The model under review builds one solid part; all positions refer to its coordinate system, in mm. Face numbers are marked on the shaded views. A direction names the side the tool comes from. Give positions to 0.01 mm unless a question says otherwise; leave off trailing zeros. Order: outer loops, then holes, each group sorted by start corner. A loop starts at its lowest first (then second) coordinate and runs counter-clockwise, first axis right, second up. Notation, with made-up numbers: (62, 12.5) - (113, 12.5) arc R31 ccw to (113, 41.5) - close; hole circle Ø5 at (50.25, -29). An arc over 180 degrees is marked (long way). Write item = value, one per line. Start each with the question number.
1. We need section B-B, the plane z = 0. Give the boundary of the cut face in (x, y).
2. Machinability: for the marked faces 1 and 2, which of the approach directions +Z, -Z, +X, -X, +Y, -Y give a long, thin tool a straight path to every point of the face, cutting with its end or side? Answer none if there is none.
3. We need section A-A, the plane x = 0. Give the boundary of the cut face in (y, z), and give its area (3 significant figures).
4. Wall thickness on probe 1 along X at (y, z) = (25.5, 0); probe 2 along Y at (x, z) = (-9, -9); probe 3 along X at (y, z) = (4, 15): over which ranges is each line inside the solid? List them lowest first.
5. We need section C-C, the plane y = 27. Give the boundary of the cut face in (x, z).
6. For P1, Ø5.5, axis at x = 0, z = 15, coming from the +Y side; P2, Ø8, axis at y = 18, z = -6.5, coming from the +X side; P3, Ø4, axis at y = 17.5, z = 5.5, coming from the -X side; P4, Ø10, axis at y = 15, z = 2, coming from the +X side, all flat-tipped, find the tip position at first contact; note any pin that passes through.
7. Mouldability with a two-part tool opening along Z and no side actions: class the marked faces 3, 4, 5 and 6 as pulls with the +Z half, pulls with the -Z half, needs draft (parallel to the pull), parting line crosses it, or undercut.
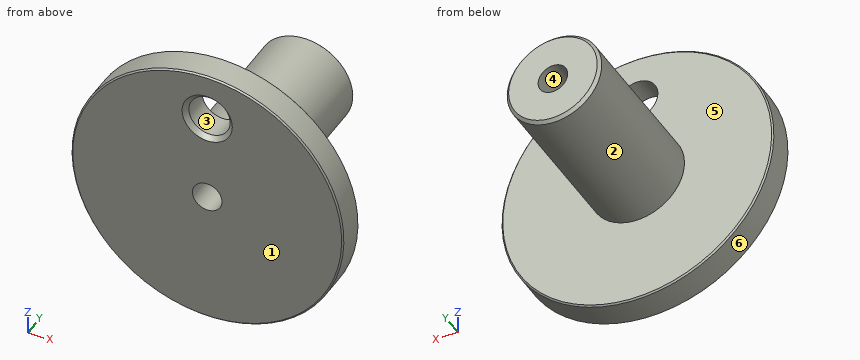
from build123d import *

# Parameters (mm, degrees)
SKETCH1_R           = 23
BOSS_EXTRUDE1_DEPTH = 32
SKETCH2_OUTSIDE_W   = 62.5
SKETCH2_OUTSIDE_H   = 62.5
SKETCH2_OUTSIDE_R   = 8
CUT_EXTRUDE1_DEPTH  = 27
SKETCH3_R           = 2.5
CUT_EXTRUDE2_DEPTH  = 46.628938186
CHAMFER1_SIZE       = 0.5
CHAMFER2_SIZE       = 0.25
SKETCH4_R           = 3.5
CUT_EXTRUDE3_DEPTH  = 46.628938186
CHAMFER3_SIZE       = 0.75


with BuildPart() as part:
    # Sketch1 → Boss-Extrude1 (new body)
    with BuildSketch(Plane(origin=(0, 0, 0), x_dir=(1, 0, 0), z_dir=(0, 1, 0))):
        with Locations(Location((0, 0, 0), (0, 0, 270))):
            Circle(SKETCH1_R)
    extrude(amount=BOSS_EXTRUDE1_DEPTH)

    # Sketch2 outside → Cut-Extrude1 (cut)
    with BuildSketch(Plane(origin=(0, 32, 0), x_dir=(1, 0, 0), z_dir=(0, 1, 0))):
        Rectangle(SKETCH2_OUTSIDE_W, SKETCH2_OUTSIDE_H)
        with Locations(Location((0, 0, 0), (0, 0, 270))):
            Circle(SKETCH2_OUTSIDE_R, mode=Mode.SUBTRACT)
    extrude(amount=-CUT_EXTRUDE1_DEPTH, mode=Mode.SUBTRACT)

    # Sketch3 → Cut-Extrude2 (cut, through all)
    with BuildSketch(Plane(origin=(0, 32, 0), x_dir=(1, 0, 0), z_dir=(0, 1, 0))):
        with Locations(Location((0, 0, 0), (0, 0, 270))):
            Circle(SKETCH3_R)
    extrude(amount=-CUT_EXTRUDE2_DEPTH, mode=Mode.SUBTRACT)

    # Chamfer1
    chamfer1_edges = [part.edges().sort_by_distance(p)[0] for p in [
        (0, 32, -8),
    ]]
    chamfer(chamfer1_edges, length=CHAMFER1_SIZE)

    # Chamfer2
    chamfer2_edges = [part.edges().sort_by_distance(p)[0] for p in [
        (0, 0, -23),
        (0, 5, -23),
    ]]
    chamfer(chamfer2_edges, length=CHAMFER2_SIZE)

    # Sketch4 → Cut-Extrude3 (cut, through all)
    with BuildSketch(Plane.XZ):
        with Locations(Location((0, 15, 0), (0, 0, 270))):
            Circle(SKETCH4_R)
    extrude(amount=-CUT_EXTRUDE3_DEPTH, mode=Mode.SUBTRACT)

    # Chamfer3
    chamfer3_edges = [part.edges().sort_by_distance(p)[0] for p in [
        (0, 0, 18.5),
    ]]
    chamfer(chamfer3_edges, length=CHAMFER3_SIZE)


solid = part.part
Model answer:
q1.outline = (-23, 0.25) - (-22.75, 0) - (-2.5, 0) - (-2.5, 32) - (-7.5, 32) - (-8, 31.5) - (-8, 5) - (-22.75, 5) - (-23, 4.75) - close; (2.5, 0) - (22.75, 0) - (23, 0.25) - (23, 4.75) - (22.75, 5) - (8, 5) - (8, 31.5) - (7.5, 32) - (2.5, 32) - close
q2.face_1 = +Z, -Z, +X, -X, -Y
q2.face_2 = +Y
q3.outline = (0, -22.75) - (0.25, -23) - (4.75, -23) - (5, -22.75) - (5, -8) - (31.5, -8) - (32, -7.5) - (32, -2.5) - (0, -2.5) - close; (0, 2.5) - (32, 2.5) - (32, 7.5) - (31.5, 8) - (5, 8) - (5, 11.5) - (0.75, 11.5) - (0, 10.75) - close; (0, 19.25) - (0.75, 18.5) - (5, 18.5) - (5, 22.75) - (4.75, 23) - (0.25, 23) - (0, 22.75) - close
q3.area = 466 mm2
q4.probe_1 = -8 to -2.5, 2.5 to 8
q4.probe_2 = 0 to 5
q4.probe_3 = -17.44 to -3.5, 3.5 to 17.44
q5.outline = circle Ø16 at (0, 0); hole circle Ø5 at (0, 0)
q6.P1 = through
q6.P2 = 7.6
q6.P3 = -7.19
q6.P4 = 8
q7.face_3 = undercut
q7.face_4 = undercut
q7.face_5 = needs draft
q7.face_6 = parting line crosses it
